```python
from build123d import *

# Parameters (mm, degrees)
SKETCH2_R           = 1.6
SKETCH2_W           = 162.5
SKETCH2_H           = 45
BOSS_EXTRUDE2_DEPTH = 4
FILLET3_R           = 3
FILLET4_R           = 5
BOSS_EXTRUDE3_DEPTH = 4
FILLET5_R           = 5
SKETCH7_W           = 12
SKETCH7_H           = 2
BOSS_EXTRUDE4_DEPTH = 12
CUT_EXTRUDE3_REACH  = 67
SKETCH8_R           = 4.25
FILLET6_R           = 5
FILLET7_R           = 3
SKETCH9_R           = 1.5
BOSS_EXTRUDE5_DEPTH = 3
FILLET8_R           = 1.5
SKETCH10_R          = 4
SKETCH10_R_2        = 1.6
BOSS_EXTRUDE6_DEPTH = 14


with BuildPart() as part:
    # Sketch2 → Boss-Extrude2 (new body)
    with BuildSketch(Plane(origin=(0, 0, 0), x_dir=(1, 0, 0), z_dir=(0, 1, 0))):
        Polygon((-93.75, -35), (-76.25, -35), (-71.25, -30), (71.25, -30), (76.25, -35), (93.75, -35), (93.75, 35), (76.25, 35), (71.25, 30), (-71.25, 30), (-76.25, 35), (-93.75, 35), align=None)
        with Locations((-85, 26.25)):
            Circle(SKETCH2_R, mode=Mode.SUBTRACT)
        with Locations((85, 26.25)):
            Circle(SKETCH2_R, mode=Mode.SUBTRACT)
        with Locations((85, -26.25)):
            Circle(SKETCH2_R, mode=Mode.SUBTRACT)
        with Locations((-85, -26.25)):
            Circle(SKETCH2_R, mode=Mode.SUBTRACT)
        Rectangle(SKETCH2_W, SKETCH2_H, mode=Mode.SUBTRACT)
    extrude(amount=BOSS_EXTRUDE2_DEPTH)

    # Fillet3
    fillet3_edges = [part.edges().sort_by_distance(p)[0] for p in [
        (-93.75, 2, -35),
        (93.75, 2, -35),
        (93.75, 2, 35),
        (-93.75, 2, 35),
    ]]
    fillet(fillet3_edges, radius=FILLET3_R)

    # Fillet4
    fillet4_edges = [part.edges().sort_by_distance(p)[0] for p in [
        (-76.25, 2, -35),
        (-71.25, 2, -30),
        (71.25, 2, -30),
        (76.25, 2, -35),
        (76.25, 2, 35),
        (71.25, 2, 30),
        (-71.25, 2, 30),
        (-76.25, 2, 35),
        (81.25, 2, -22.5),
        (-81.25, 2, -22.5),
        (-81.25, 2, 22.5),
        (81.25, 2, 22.5),
    ]]
    fillet(fillet4_edges, radius=FILLET4_R)

    # Sketch5 → Boss-Extrude3 (add)
    with BuildSketch(Plane(origin=(0, 0, 0), x_dir=(1, 0, 0), z_dir=(0, 1, 0))):
        Polygon((-26.25, -10.5), (-2, -10.5), (-2, -25.93943087), (2, -25.93943087), (2, -10.5), (26.25, -10.5), (26.25, 30), (-26.25, 30), align=None)
        with BuildLine():
            Line((-16.9, 26.25), (16.9, 26.25))
            Line((16.9, 26.25), (16.9, 23.25))
            ThreePointArc((16.9, 23.25), (17.661522369, 21.411522369), (19.5, 20.65))
            Line((19.5, 20.65), (22.5, 20.65))
            Line((22.5, 20.65), (22.5, -1.15))
            Line((22.5, -1.15), (19.5, -1.15))
            ThreePointArc((19.5, -1.15), (17.661522369, -1.911522369), (16.9, -3.75))
            Line((16.9, -3.75), (16.9, -6.75))
            Line((16.9, -6.75), (-16.9, -6.75))
            Line((-16.9, -6.75), (-16.9, -3.75))
            ThreePointArc((-16.9, -3.75), (-17.661522369, -1.911522369), (-19.5, -1.15))
            Line((-19.5, -1.15), (-22.5, -1.15))
            Line((-22.5, -1.15), (-22.5, 20.65))
            Line((-22.5, 20.65), (-19.5, 20.65))
            ThreePointArc((-19.5, 20.65), (-17.661522369, 21.411522369), (-16.9, 23.25))
            Line((-16.9, 23.25), (-16.9, 26.25))
        make_face(mode=Mode.SUBTRACT)
    extrude(amount=BOSS_EXTRUDE3_DEPTH)

    # Fillet5
    fillet5_edges = [part.edges().sort_by_distance(p)[0] for p in [
        (-26.25, 2, -22.5),
        (26.25, 2, -22.5),
        (26.25, 2, 10.5),
        (-26.25, 2, 10.5),
    ]]
    fillet(fillet5_edges, radius=FILLET5_R)

    # Sketch7 → Boss-Extrude4 (add)
    with BuildSketch(Plane(origin=(0, 4, 0), x_dir=(1, 0, 0), z_dir=(0, 1, 0))):
        with Locations((-63.178932188, 29)):
            Rectangle(SKETCH7_W, SKETCH7_H)
    extrude(amount=BOSS_EXTRUDE4_DEPTH)

    # Sketch8 → Cut-Extrude3 (cut, up to next)
    with BuildSketch(Plane(origin=(0, 0, -30), x_dir=(-1, 0, 0), z_dir=(0, 0, -1)), mode=Mode.PRIVATE) as cut_extrude3_sk1:
        with Locations((63.178932188, 10)):
            Circle(SKETCH8_R)
    cut_extrude3_tool1 = extrude(cut_extrude3_sk1.sketch, amount=-CUT_EXTRUDE3_REACH, mode=Mode.PRIVATE) & part.part
    add(cut_extrude3_tool1.solids().sort_by_distance((-63.178932, 10, -30))[0], mode=Mode.SUBTRACT)

    # Fillet6
    fillet6_edges = [part.edges().sort_by_distance(p)[0] for p in [
        (-57.178932188, 4, -29),
        (-69.178932188, 16, -29),
        (-57.178932188, 16, -29),
    ]]
    fillet(fillet6_edges, radius=FILLET6_R)

    # Fillet7
    fillet7_edges = [part.edges().sort_by_distance(p)[0] for p in [
        (2, 2, 22.5),
        (-2, 2, 22.5),
        (-2, 2, 10.5),
        (2, 2, 10.5),
    ]]
    fillet(fillet7_edges, radius=FILLET7_R)

    # Sketch9 → Boss-Extrude5 (add)
    with BuildSketch(Plane(origin=(0, 4, 0), x_dir=(1, 0, 0), z_dir=(0, 1, 0))):
        with Locations((-19.5, -3.75)):
            Circle(SKETCH9_R)
        with Locations((-19.5, 23.25)):
            Circle(SKETCH9_R)
        with Locations((19.5, 23.25)):
            Circle(SKETCH9_R)
        with Locations((19.5, -3.75)):
            Circle(SKETCH9_R)
    extrude(amount=BOSS_EXTRUDE5_DEPTH)

    # Fillet8
    fillet8_edges = [part.edges().sort_by_distance(p)[0] for p in [
        (-21, 7, 3.75),
        (-21, 7, -23.25),
        (18, 7, -23.25),
        (18, 7, 3.75),
    ]]
    fillet(fillet8_edges, radius=FILLET8_R)

    # Sketch10 → Boss-Extrude6 (add)
    with BuildSketch(Plane(origin=(0, 4, 0), x_dir=(1, 0, 0), z_dir=(0, 1, 0))):
        with Locations((-85, 26.25)):
            Circle(SKETCH10_R)
        with Locations((-85, 26.25)):
            Circle(SKETCH10_R_2, mode=Mode.SUBTRACT)
        with Locations((85, 26.25)):
            Circle(SKETCH10_R)
        with Locations((85, 26.25)):
            Circle(SKETCH10_R_2, mode=Mode.SUBTRACT)
        with Locations((85, -26.25)):
            Circle(SKETCH10_R)
        with Locations((85, -26.25)):
            Circle(SKETCH10_R_2, mode=Mode.SUBTRACT)
        with Locations((-85, -26.25)):
            Circle(SKETCH10_R)
        with Locations((-85, -26.25)):
            Circle(SKETCH10_R_2, mode=Mode.SUBTRACT)
    extrude(amount=BOSS_EXTRUDE6_DEPTH)


solid = part.part
```
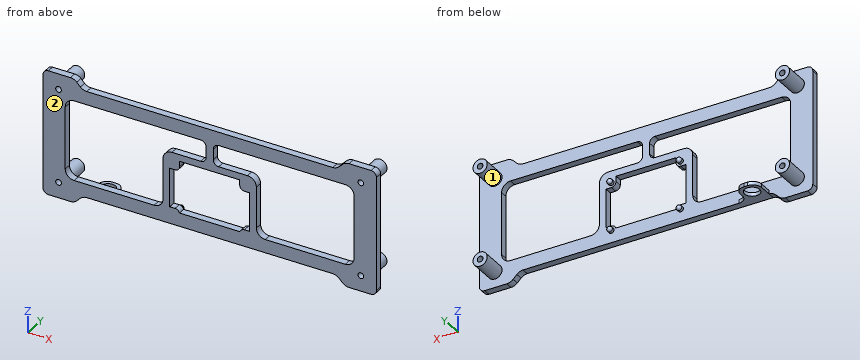
Part model, mm, in its own coordinate system. Face numbers are marked on the shaded views. Round coordinates to 2 decimals unless told otherwise and drop trailing zeros. Loops run counter-clockwise (first coordinate to the right, second up) from the corner with the lowest first, then second, coordinate; pieces in that order, holes last. Notation, with made-up numbers: (43.25, 83.25) -> (53.25, 83.25) arc R6 cw to (53.25, 87.25) -> close; hole circle Ø5 at (-14.5, 24). An arc over 180 degrees is marked (long way). Use a Markdown table: item, result.
1) Cut at A-A, the plane x = 53. List the corners of the cut face in (y, z), and give its area (3 significant figures).
The answers:
| item | result |
|---|---|
| outline | (0, -30) -> (4, -30) -> (4, -22.5) -> (0, -22.5) -> close; (0, 22.5) -> (4, 22.5) -> (4, 30) -> (0, 30) -> close |
| area | 60.0 mm2 |
2) Cut at B-B, the plane y = 2. State how many separate pieces and enclosed holes the cut face has, and give its area (3 significant figures).
The answers:
| item | result |
|---|---|
| separate pieces | 1 |
| enclosed holes | 7 |
| area | 4,870 mm2 |
3) Pull direction Z, two halves, no side cores. Call the marked faces 1 and 2: pulls with the +Z half, pulls with the -Z half, needs draft (parallel to the pull), parting line crosses it, or undercut.
The answers:
| item | result |
|---|---|
| face 1 | undercut |
| face 2 | needs draft |
4) Drop flat-ended pins along their axis: pin 1 Ø4 at (x, y) = (39.5, 6.5) entering from -Z; pin 2 Ø3 at (x, y) = (-26, 1.5) entering from +Z; pin 3 Ø4 at (y, z) = (15, 25) entering from +X; pin 4 Ø3.5 at (x, y) = (-57.5, 8) entering from +Z. Give the stop position or say it passes through.
The answers:
| item | result |
|---|---|
| pin 1 | passes through |
| pin 2 | stops at z = 30 |
| pin 3 | stops at x = 89 |
| pin 4 | stops at z = -28 |
5) Probe line 1 (X direction, y = 12.75, z = 26.25); line 2 (Z direction, x = -85, y = 8); line 3 (X direction, y = 3.25, z = -16). List the from-to ranges inside material, lowest first. Write a range as [from, to].
The answers:
| item | result |
|---|---|
| line 1 | x = [-89, -86.6], [-83.4, -81], [81, 83.4], [86.6, 89] |
| line 2 | z = [-30.25, -27.85], [-24.65, -22.25], [22.25, 24.65], [27.85, 30.25] |
| line 3 | x = [-93.75, -81.25], [-26.25, -22.5], [22.5, 26.25], [81.25, 93.75] |
